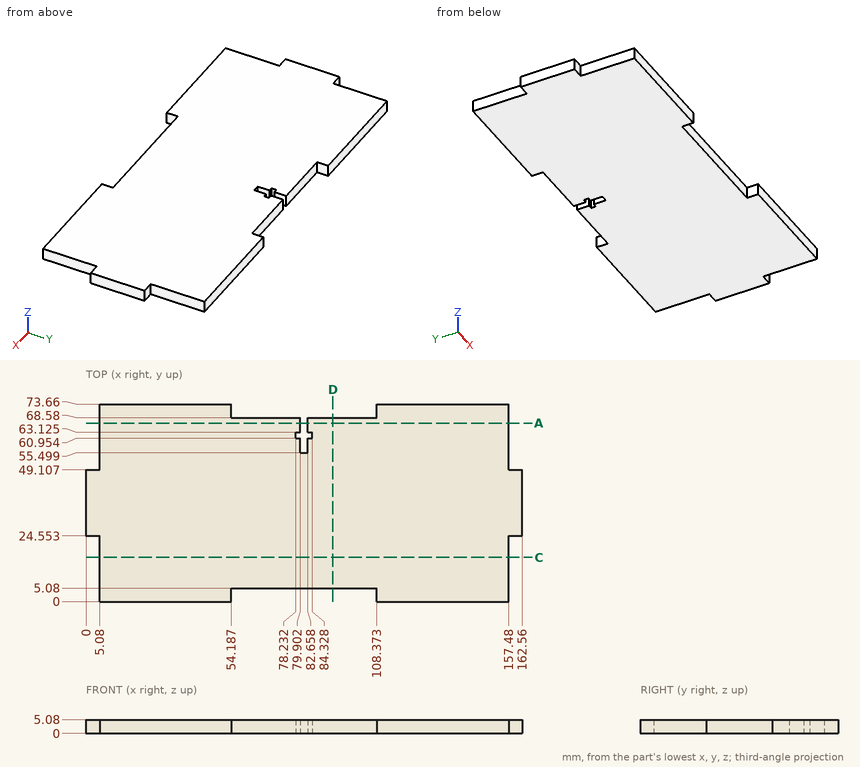
Input: dimensioned drawing with shaded views. Units: mm. Origin: part minimum x, y, z. Coordinates: 2 decimals unless noted, no trailing zeros. Order: outer loops, then holes, each group sorted by start corner. A loop starts at its lowest first (then second) coordinate and runs counter-clockwise, first axis right, second up. Notation, with made-up numbers: M 27,4.25 L 34,4.25 A26 cw 34,31.25 Z; hole C -28.5,20.25 d9. An arc over 180 degrees is marked long. Write each question's results on one line, items separated by ' | '. Start each with the question number.
Item 1: First-contact query: pin 1 Ø1.8 at (x, z) = (83.5, 2.5) entering from -Y; pin 2 Ø1.5 at (y, z) = (66, 1.5) entering from -X; pin 3 Ø2.5 at (y, z) = (61, 3.5) entering from +X. Flat tips, straight axial feed; report the tip coordinate or a pass-through.
Item 2: Cut plane A-A (y = 66.5). Return loops of the section in (x, z), and give its area (3 significant figures).
Item 3: Cut plane D-D (x = 92). Return loops of the section in (y, z).
Item 4: Cut plane C-C (y = 16.5). Return loops of the section in (x, z).
Item 5: Line query: probe 1 along X at (y, z) = (60.5, 4.4); probe 2 along X at (y, z) = (24.5, 4.45); probe 3 along Y at (x, z) = (81.5, 0.35). Output: solid intervals per line, ascending.
Checked values:
1) pin 1: stops at y = 5.08 | pin 2: stops at x = 5.08 | pin 3: stops at x = 157.48
2) outline: M 5.08,0 L 79.9,0 L 79.9,5.08 L 5.08,5.08 Z; M 82.66,0 L 157.48,0 L 157.48,5.08 L 82.66,5.08 Z | area: 760 mm2
3) outline: M 5.08,0 L 68.58,0 L 68.58,5.08 L 5.08,5.08 Z
4) outline: M 5.08,0 L 157.48,0 L 157.48,5.08 L 5.08,5.08 Z
5) probe 1: x = 5.08 to 79.9, 82.66 to 157.48 | probe 2: x = 5.08 to 157.48 | probe 3: y = 5.08 to 55.5
